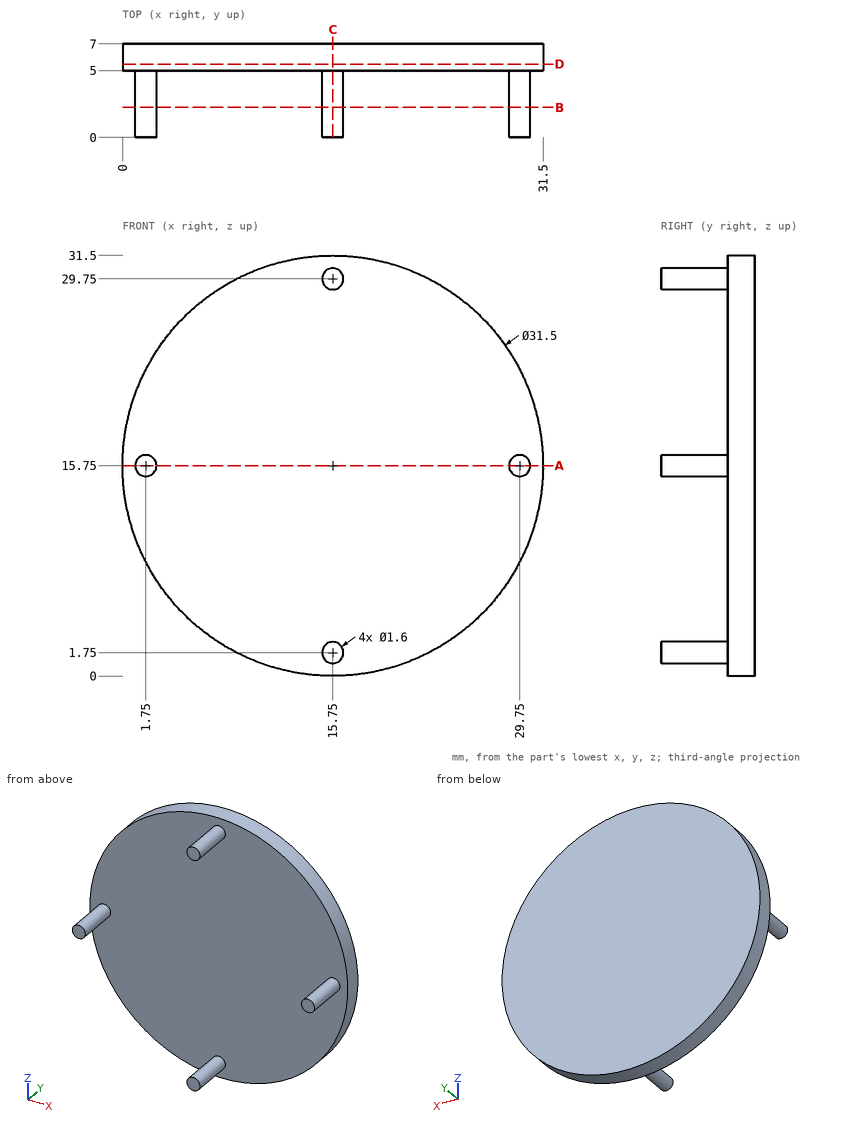
Drawing for the job (mm, zero at the part's lowest x, y, z). Coordinates: 2 decimals unless noted, no trailing zeros. Order: outer loops, then holes, each group sorted by start corner. A loop starts at its lowest first (then second) coordinate and runs counter-clockwise, first axis right, second up. Notation, with made-up numbers: (35, 72) -> (79, 72) arc R20 cw to (79, 78) -> close; hole circle Ø8 at (-8, -14.5). An arc over 180 degrees is marked (long way). Return JSON: item names as keys, results as strings.
Item 1: Wall check: line 1 along Y through (x, z) = (10, 19.5); line 2 along X through (y, z) = (6.5, 11); line 3 along Z through (x, y) = (5.5, 5.5). Give the ranges that are in metal, low to high. Write a range as from..to.
Model answer:
{"line 1": "y = 5..7", "line 2": "x = 0.73..30.77", "line 3": "z = 3.79..27.71"}
Item 2: Slice it at C-C (x = 15.75). Write the cut outline in (y, z).
Model answer:
{"outline": "(0, 0.95) -> (5, 0.95) -> (5, 0) -> (7, 0) -> (7, 31.5) -> (5, 31.5) -> (5, 30.55) -> (0, 30.55) -> (0, 28.95) -> (5, 28.95) -> (5, 2.55) -> (0, 2.55) -> close"}
Item 3: Slice it at D-D (y = 5.5). Write the cut outline in (x, z).
Model answer:
{"outline": "circle Ø31.5 at (15.75, 15.75)"}
Item 4: Slice it at A-A (z = 15.75). Write the cut outline in (x, y), then the cut area to 3 significant figures.
Model answer:
{"outline": "(0, 5) -> (0.95, 5) -> (0.95, 0) -> (2.55, 0) -> (2.55, 5) -> (28.95, 5) -> (28.95, 0) -> (30.55, 0) -> (30.55, 5) -> (31.5, 5) -> (31.5, 7) -> (0, 7) -> close", "area": "79.0 mm²"}
Item 5: Pin check, flat tips, straight feed: P1, Ø6, axis at x = 7, z = 17, coming from the -Y side; P2, Ø2, axis at x = 7, y = 5.5, coming from the +Z side; P3, Ø1, axis at y = 2.5, z = 16.5, coming from the -X side. Stop position of each tip, or through.
Model answer:
{"P1": "stops at y = 5", "P2": "stops at z = 29.46", "P3": "stops at x = 0.99"}
Item 6: Slice it at B-B (y = 2.25). Write the cut outline in (x, z).
Model answer:
{"outline": "circle Ø1.6 at (1.75, 15.75); circle Ø1.6 at (15.75, 1.75); circle Ø1.6 at (15.75, 29.75); circle Ø1.6 at (29.75, 15.75)"}
